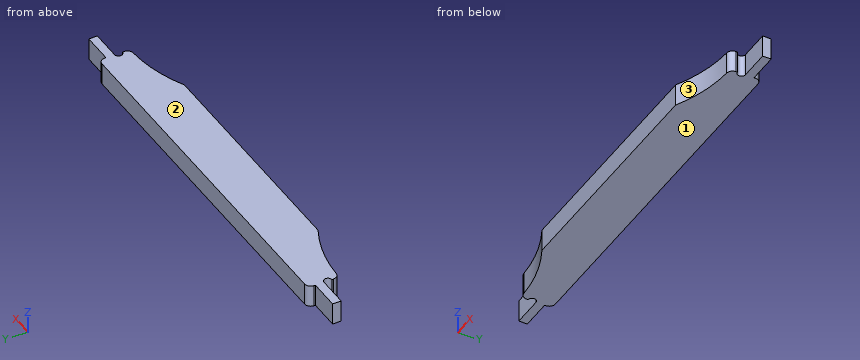
```python
from build123d import *

# Parameters (mm, degrees)
F1_DEPTH = 18
F2_R     = 5
F4_DEPTH = 18.001
F5_R     = 5


with BuildPart() as f1:
    # F0 (on Top) → F1 (new body)
    with BuildSketch(Plane.XY):
        with BuildLine():
            Line((-177, 7), (-177, 0))
            Line((-177, 0), (-152, 0))
            Line((-152, 0), (-152, -12.5))
            ThreePointArc((-152, -12.5), (-123.683706, -15.924358), (-97, -26))
            Line((-97, -26), (0, -26))
            Line((0, -26), (97, -26))
            ThreePointArc((97, -26), (123.683706, -15.924358), (152, -12.5))
            Line((152, -12.5), (152, 0))
            Line((152, 0), (177, 0))
            Line((177, 0), (177, 7))
            Line((177, 7), (152, 7))
            Line((152, 7), (152, 13))
            Line((152, 13), (0, 13))
            Line((0, 13), (-152, 13))
            Line((-152, 13), (-152, 7))
            Line((-152, 7), (-177, 7))
        make_face()
    extrude(amount=F1_DEPTH)

    # F2
    f2_edges = [f1.edges().sort_by_distance(p)[0] for p in [
        (-152, -12.5, 9),
        (152, -12.5, 9),
    ]]
    fillet(f2_edges, radius=F2_R)

    # F3 (on face) → F4 (cut, through all)
    with BuildSketch(Plane.XY.offset(18)):
        with BuildLine():
            ThreePointArc((152, 0), (148.825, -3.175), (152, -6.35))
            Line((152, -6.35), (152, 0))
        make_face()
        with BuildLine():
            Line((-152, 0), (-152, -6.36))
            ThreePointArc((-152, -6.36), (-148.82, -3.18), (-152, 0))
        make_face()
    extrude(amount=-F4_DEPTH, mode=Mode.SUBTRACT)

    # F5
    f5_edges = [f1.edges().sort_by_distance(p)[0] for p in [
        (-152, 13, 9),
        (152, 13, 9),
    ]]
    fillet(f5_edges, radius=F5_R)


solid = f1.part
```
Input: part model. Units: mm. Frame: model coordinates. Face numbers are marked on the shaded views. Coordinates: 2 decimals unless noted, no trailing zeros. Order: outer loops, then holes, each group sorted by start corner. A loop starts at its lowest first (then second) coordinate and runs counter-clockwise, first axis right, second up. Notation, with made-up numbers: (-8.5, 24.25) - (19.5, 24.25) arc R20 ccw to (19.5, 56.25) - close; hole circle Ø3 at (37, 59). An arc over 180 degrees is marked (long way). Return JSON: item names as keys, results as strings.
Q1. Cut plane C-C (x = 107.5). Return loops of the section in (y, z), then the cut area to 3 significant figures.
The answers:
{"outline": "(-21.15, 0) - (13, 0) - (13, 18) - (-21.15, 18) - close", "area": "615 mm2"}
Q2. Draft query along Z for the marked faces 1, 2 and 3. Return one class per face: +Z half, -Z half, draft (parallel to the pull), parting line (faces both ways), or undercut.
The answers:
{"face 1": "-Z half", "face 2": "+Z half", "face 3": "draft"}
Q3. Cut plane B-B (y = -3.18). Return loops of the section in (x, z) (3 decimals), then the cut area to 3 significant figures.
The answers:
{"outline": "(-148.82, 0) - (148.825, 0) - (148.825, 18) - (-148.82, 18) - close", "area": "5,360 mm2"}
Q4. Ray query, probe 1 along X at (y, z) = (8.5, 8); probe 2 along Y at (x, z) = (-147, 4.5); probe 3 along X at (y, z) = (10, 6). Return the intervals inside material, ascending.
The answers:
{"probe 1": "x = -151.97 to 151.97", "probe 2": "y = -12.61 to 13", "probe 3": "x = -151.58 to 151.58"}
Q5. Cut plane A-A (z = 10.25). Return loops of the section in (x, y) (3 decimals).
The answers:
{"outline": "(-177, 0) - (-152, 0) arc R3.18 cw to (-152, -6.36) - (-152, -7.601) arc R5 ccw to (-147.202, -12.597) arc R118.787 cw to (-97, -26) - (97, -26) arc R118.787 cw to (147.202, -12.597) arc R5 ccw to (152, -7.601) - (152, -6.35) arc R3.175 cw to (152, 0) - (177, 0) - (177, 7) - (152, 7) - (152, 8) arc R5 ccw to (147, 13) - (-147, 13) arc R5 ccw to (-152, 8) - (-152, 7) - (-177, 7) - close"}
Q6. First-contact query: pin 1 (1 mm diameter, centred on y = -7, z = 5, fed in from -X); pin 2 (9 mm diameter, centred on x = 160.5, z = 12.5, fed in from -Y); pin 3 (5.5 mm diameter, centred on x = -163, z = 11.5, fed in from +Y). Flat tips, straight axial feed; report the tip coordinate or a pass-through.
The answers:
{"pin 1": "stops at x = -152", "pin 2": "stops at y = 0", "pin 3": "stops at y = 7"}
